```python
from build123d import *

# Parameters (mm, degrees)
SKETCH1_R           = 4.25
BOSS_EXTRUDE1_DEPTH = 12.7
SKETCH3_R           = 4.25
BOSS_EXTRUDE3_DEPTH = 12.7
SKETCH2_R           = 4.25
BOSS_EXTRUDE2_DEPTH = 6.35


with BuildPart() as part:
    # Sketch1 → Boss-Extrude1 (new body)
    with BuildSketch(Plane.XY):
        with BuildLine():
            Line((93.98, -12.7), (-93.98, -12.7))
            ThreePointArc((-93.98, -12.7), (-96.674076836, -11.584076836), (-97.79, -8.89))
            Line((-97.79, -8.89), (-97.79, 8.89))
            ThreePointArc((-97.79, 8.89), (-96.674076836, 11.584076836), (-93.98, 12.7))
            Line((-93.98, 12.7), (93.98, 12.7))
            ThreePointArc((93.98, 12.7), (96.674076836, 11.584076836), (97.79, 8.89))
            Line((97.79, 8.89), (97.79, -8.89))
            ThreePointArc((97.79, -8.89), (96.674076836, -11.584076836), (93.98, -12.7))
        make_face()
        with Locations((-88.9, 0)):
            Circle(SKETCH1_R, mode=Mode.SUBTRACT)
        with Locations((88.9, 0)):
            Circle(SKETCH1_R, mode=Mode.SUBTRACT)
    extrude(amount=BOSS_EXTRUDE1_DEPTH)

    # Sketch3 → Boss-Extrude3 (add, through all)
    with BuildSketch(Plane.XY.offset(12.7)):
        with BuildLine():
            Line((-6.335384206, -97.155), (6.335384206, -97.155))
            ThreePointArc((6.335384206, -97.155), (9.927486654, -95.667102448), (11.415384206, -92.075))
            Line((11.415384206, -92.075), (11.415384206, 92.075))
            ThreePointArc((11.415384206, 92.075), (9.927486654, 95.667102448), (6.335384206, 97.155))
            Line((6.335384206, 97.155), (-6.335384206, 97.155))
            ThreePointArc((-6.335384206, 97.155), (-9.927486654, 95.667102448), (-11.415384206, 92.075))
            Line((-11.415384206, 92.075), (-11.415384206, -92.075))
            ThreePointArc((-11.415384206, -92.075), (-9.927486654, -95.667102448), (-6.335384206, -97.155))
        make_face()
        with Locations((0, 88.9)):
            Circle(SKETCH3_R, mode=Mode.SUBTRACT)
        with Locations((0, -88.9)):
            Circle(SKETCH3_R, mode=Mode.SUBTRACT)
    extrude(amount=-BOSS_EXTRUDE3_DEPTH)

    # Sketch2 → Boss-Extrude2 (add)
    with BuildSketch(Plane(origin=(0, 0, 0), x_dir=(-1, 0, 0), z_dir=(0, 0, -1))):
        with Locations(Location((0, 88.9, 0), (0, 0, 180))):
            Circle(SKETCH2_R)
        with Locations((-88.9, 0)):
            Circle(SKETCH2_R)
        with Locations(Location((0, -88.9, 0), (0, 0, 180))):
            Circle(SKETCH2_R)
        with Locations((88.9, 0)):
            Circle(SKETCH2_R)
    extrude(amount=-BOSS_EXTRUDE2_DEPTH)


solid = part.part
```
Input: part model. Units: mm. Frame: model coordinates. A direction names the side the tool comes from. Coordinates: 2 decimals unless noted, no trailing zeros. Loops run counter-clockwise (first coordinate to the right, second up) from the corner with the lowest first, then second, coordinate; pieces in that order, holes last. Notation, with made-up numbers: M 70.25,-6.75 L 101.25,-6.75 A21 ccw 101.25,14.25 Z; hole C 27.25,88 d11. An arc over 180 degrees is marked long. Use a Markdown table: item, result. Add a question column.
1) Draft query along X for faces 1 (the cylindrical face through (-89.453, 4.214, 9.481)), 2 (the flat face through (-53, 12.7, 6)), 3 (the flat face through (-11.415, -52, 6)). Return one class per face: +X half, -X half, draft (parallel to the pull), parting line (faces both ways), or undercut.
2) Pin query (flat end, axial travel): P1, Ø6.5, axis at y = -61.5, z = 5, coming from the +X side; P2, Ø2.5, axis at x = -1, y = 90.5, coming from the +Z side; P3, Ø6.5, axis at x = -62.5, z = 4.5, coming from the -Y side. Return the tip coordinate at first contact, or that it passes through.
3) Section A-A, the plane x = 0. Return the cut outline in (y, z) (3 decimals), plus the area to 3 significant figures.
4) Section B-B, the plane z = 8.5. Return the cut outline in (x, y) (3 decimals), plus the area to 3 significant figures.
5) Section D-D, the plane x = -88.9. Return the cut outline in (y, z), plus the area to 3 significant figures.
6) Section C-C, the plane y = 0. Return the cut outline in (x, z).
7) Set-up query: faces 4 (the flat face through (-11.415, 53, 6)), 5 (the flat face through (11.415, 52, 6)), 6 (the flat face through (53, -12.7, 6)), 7 (the flat face through (0, -89, 6.35)). Return all of +Z, -Z, +X, -X, +Y, -Y with unobstructed straight access to the full face (end or side cutting, diameter ignored); none if empty.
8) Line query: L1, parallel to X at y = 0, z = 10; L2, parallel to Y at x = 0, z = 9.25 (3 decimals); L3, parallel to Y at x = -88.9, z = 8. Output: solid intervals per line, ascending. Write a range as from..to.
Answer below:
| question | item | result |
|---|---|---|
| 1 | face 1 | undercut |
| 1 | face 2 | draft |
| 1 | face 3 | -X half |
| 2 | P1 | x = 11.42 |
| 2 | P2 | z = 6.35 |
| 2 | P3 | y = -12.7 |
| 3 | outline | M -97.155,0 L 97.155,0 L 97.155,12.7 L 93.15,12.7 L 93.15,6.35 L 84.65,6.35 L 84.65,12.7 L -84.65,12.7 L -84.65,6.35 L -93.15,6.35 L -93.15,12.7 L -97.155,12.7 Z |
| 3 | area | 2,360 mm2 |
| 4 | outline | M -97.79,-8.89 A3.81 ccw -93.98,-12.7 L -11.415,-12.7 L -11.415,-92.075 A5.08 ccw -6.335,-97.155 L 6.335,-97.155 A5.08 ccw 11.415,-92.075 L 11.415,-12.7 L 93.98,-12.7 A3.81 ccw 97.79,-8.89 L 97.79,8.89 A3.81 ccw 93.98,12.7 L 11.415,12.7 L 11.415,92.075 A5.08 ccw 6.335,97.155 L -6.335,97.155 A5.08 ccw -11.415,92.075 L -11.415,12.7 L -93.98,12.7 A3.81 ccw -97.79,8.89 Z; hole C -88.9,0 d8.5; hole C 0,-88.9 d8.5; hole C 0,88.9 d8.5; hole C 88.9,0 d8.5 |
| 4 | area | 8,560 mm2 |
| 5 | outline | M -12.7,0 L 12.7,0 L 12.7,12.7 L 4.25,12.7 L 4.25,6.35 L -4.25,6.35 L -4.25,12.7 L -12.7,12.7 Z |
| 5 | area | 269 mm2 |
| 6 | outline | M -97.79,0 L 97.79,0 L 97.79,12.7 L 93.15,12.7 L 93.15,6.35 L 84.65,6.35 L 84.65,12.7 L -84.65,12.7 L -84.65,6.35 L -93.15,6.35 L -93.15,12.7 L -97.79,12.7 Z |
| 7 | face 4 | +Z, -Z, -X, +Y |
| 7 | face 5 | +Z, -Z, +X, +Y |
| 7 | face 6 | +Z, -Z, +X, -Y |
| 7 | face 7 | +Z |
| 8 | L1 | -97.79..-93.15, -84.65..84.65, 93.15..97.79 |
| 8 | L2 | -97.155..-93.15, -84.65..84.65, 93.15..97.155 |
| 8 | L3 | -12.7..-4.25, 4.25..12.7 |
